Print and shaded views of the part. All mm, measured from the part's lowest x, y and z. Give positions to 0.01 mm unless a question says otherwise; leave off trailing zeros. Write each loop counter-clockwise with the first axis right and the second up, starting at its lowest first coordinate (ties: lowest second). Pieces come first, ordered by that corner, then holes. Notation, with made-up numbers: M -23,-8.75 L 32,-8.75 A20 ccw 32,16.25 Z; hole C -21.5,-38.75 d11. An arc over 180 degrees is marked long. One line per question, with ' | ' between items. Start each with the question number.
1. Cut at A-A, the plane y = 35. Count the separate pieces of the cut face and the enclosed holes in it, then the cut area to 3 significant figures.
2. Cut at B-B, the plane y = 61.5. Write the cut outline in (x, z) (1 decimal).
3. Wall check: L1, parallel to X at y = 66, z = 2.9 (1 decimal); L2, parallel to Y at x = 47.5, z = 0.2 (1 decimal); L3, parallel to X at y = 63, z = 2.4 (1 decimal). Give the ranges that are in metal, low to high.
4. Cut at D-D, the plane y = 52.5. Write the cut outline in (x, z) (1 decimal), then the cut area to 3 significant figures.
5. Flat gauge pins, fed straight in: pin 1 (1 mm diameter, centred on y = 57, z = 1, fed in from +X) (1 decimal); pin 2 (1.8 mm diameter, centred on x = 1.59, y = 35, fed in from -Z); pin 3 (1 mm diameter, centred on y = 59, z = 2, fed in from -X) (1 decimal); pin 4 (0.5 mm diameter, centred on x = 40.5, z = 2, fed in from +Y) (1 decimal). Where does each tip first touch, or does it go through?
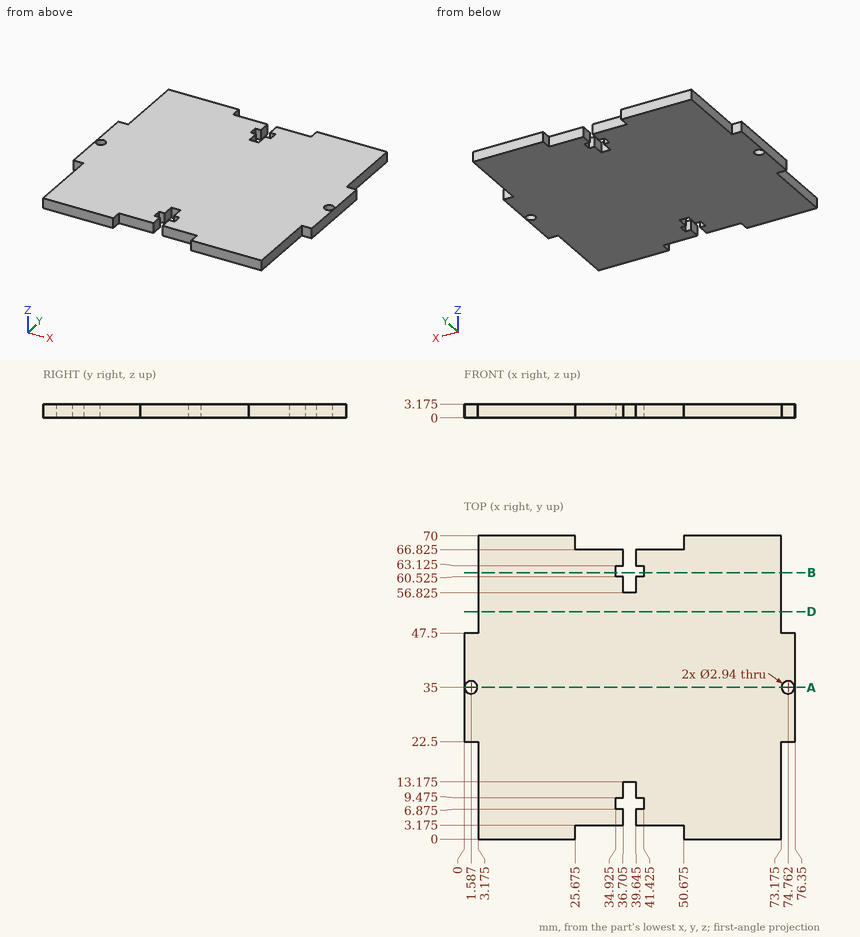
Here are the results:
1) separate pieces: 3 | enclosed holes: 0 | area: 224 mm^2
2) outline: M 3.2,0 L 34.9,0 L 34.9,3.2 L 3.2,3.2 Z; M 41.4,0 L 73.2,0 L 73.2,3.2 L 41.4,3.2 Z
3) L1: 3.2 to 36.7, 39.6 to 73.2 | L2: 3.2 to 66.8 | L3: 3.2 to 34.9, 41.4 to 73.2
4) outline: M 3.2,0 L 73.2,0 L 73.2,3.2 L 3.2,3.2 Z | area: 222 mm^2
5) pin 1: x = 73.2 | pin 2: through | pin 3: x = 3.2 | pin 4: y = 66.8
